Can you work these out from the drawing? Everything is in mm from the part's minimum corner. A direction names the side the tool comes from. Give positions to 0.01 mm unless a question says otherwise; leave off trailing zeros. Loops run counter-clockwise (first coordinate to the right, second up) from the corner with the lowest first, then second, coordinate; pieces in that order, holes last. Notation, with made-up numbers: (54, 38.25) -> (108, 38.25) arc R9 cw to (108, 45.25) -> close; hole circle Ø4 at (41, -14.5). An arc over 180 degrees is marked (long way). Return JSON: item names as keys, results as strings. Group by question number.
Q1. Will these pins go through, and if not, where does the flat tip stop? pin 1 (8 mm diameter, centred on x = 35, z = 38.1, fed in from -Y); pin 2 (2 mm diameter, centred on y = 39.5, z = 14.5, fed in from +X).
Q2. Suppose I cut it at A-A, the plane x = 37.5. Please give me the cut outline in (y, z).
Q3. Suppose I cut it at C-C, the plane y = 30. Please give me the cut outline in (x, z).
Q4. Which directions (+Z, -Z, +X, -X, +Y, -Y) give clear straight access to the entire face, cutting with the end or side of a thin tool? Please do the marked faces 1 and 2.
Q5. Thinking about a two-plate mould opening in Y: for the marked faces 3, 4 and 5, which applies, pulls with the +Y half, pulls with the -Y half, needs draft (parallel to the pull), parting line crosses it, or undercut?
Q6. Suppose I cut it at D-D, the plane z = 19. Please give me the cut outline in (x, y).
Q7. I need wall thicknesses on line 1 along Y through (x, z) = (21, 41); line 2 along Z through (x, y) = (35, 3); line 3 along X through (y, z) = (58, 38). Which ranges of each line are inside material? Lowest first, please. Write a range as [from, to].
Q8. Suppose I cut it at B-B, the plane z = 38.1. Please give me the cut outline in (x, y).
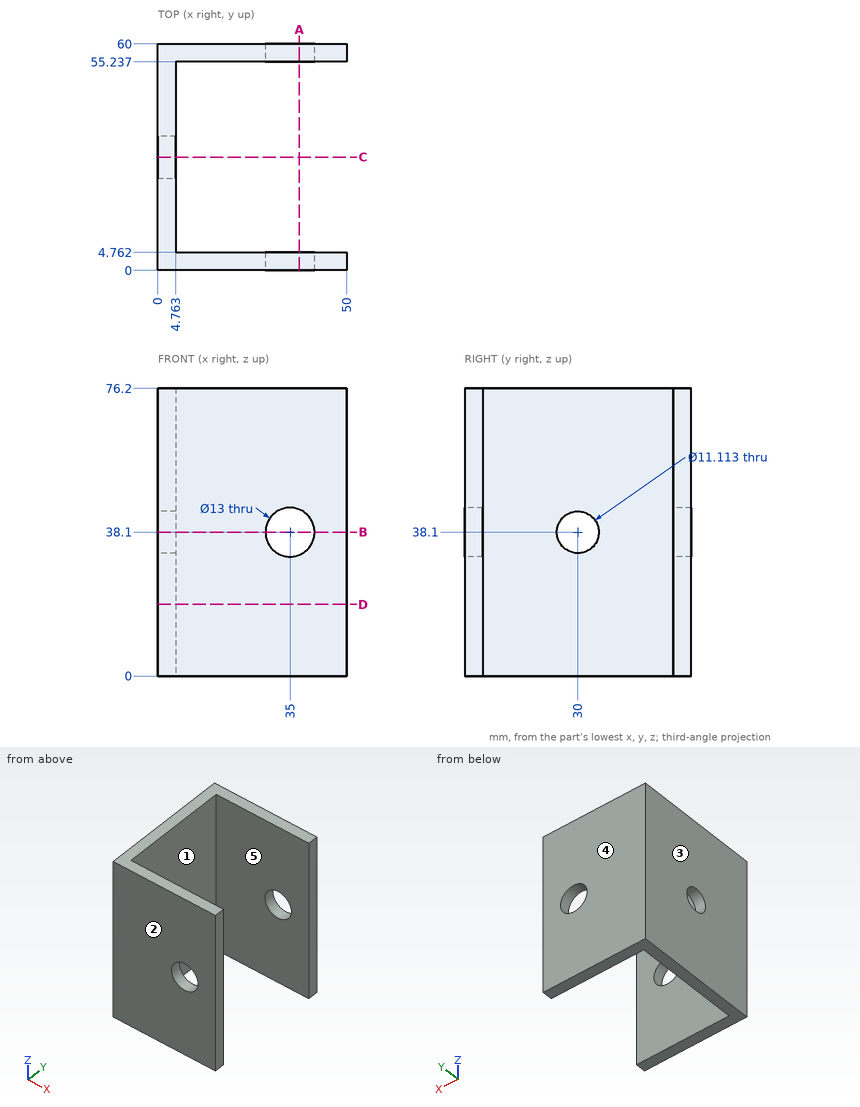
Ans:
{
 "1": {"pin 1": "passes through", "pin 2": "stops at x = 4.76"},
 "2": {"outline": "(0, 0) -> (4.76, 0) -> (4.76, 32.1) -> (0, 32.1) -> close; (0, 44.1) -> (4.76, 44.1) -> (4.76, 76.2) -> (0, 76.2) -> close; (55.24, 0) -> (60, 0) -> (60, 32.1) -> (55.24, 32.1) -> close; (55.24, 44.1) -> (60, 44.1) -> (60, 76.2) -> (55.24, 76.2) -> close"},
 "3": {"outline": "(0, 0) -> (4.76, 0) -> (4.76, 32.54) -> (0, 32.54) -> close; (0, 43.66) -> (4.76, 43.66) -> (4.76, 76.2) -> (0, 76.2) -> close"},
 "4": {"face 1": "+Z, -Z, +X", "face 2": "+Z, -Z, +X, -X, -Y"},
 "5": {"face 3": "needs draft", "face 4": "pulls with the +Y half", "face 5": "undercut"},
 "6": {"outline": "(0, 0) -> (50, 0) -> (50, 4.76) -> (4.76, 4.76) -> (4.76, 55.24) -> (50, 55.24) -> (50, 60) -> (0, 60) -> close"},
 "7": {"line 1": "y = [0, 4.76], [55.24, 60]", "line 2": "z = [0, 31.6], [44.6, 76.2]", "line 3": "x = [0, 28.5], [41.5, 50]"},
 "8": {"outline": "(0, 0) -> (28.5, 0) -> (28.5, 4.76) -> (4.76, 4.76) -> (4.76, 24.44) -> (0, 24.44) -> close; (0, 35.56) -> (4.76, 35.56) -> (4.76, 55.24) -> (28.5, 55.24) -> (28.5, 60) -> (0, 60) -> close; (41.5, 0) -> (50, 0) -> (50, 4.76) -> (41.5, 4.76) -> close; (41.5, 55.24) -> (50, 55.24) -> (50, 60) -> (41.5, 60) -> close"}
}
